The drawing under review shows one solid part. Ordinate dimensions are in mm from its lowest x, y, z. A direction names the side the tool comes from. Coordinates: 2 decimals unless noted, no trailing zeros. Order: outer loops, then holes, each group sorted by start corner. A loop starts at its lowest first (then second) coordinate and runs counter-clockwise, first axis right, second up. Notation, with made-up numbers: (39.5, 19) -> (97.5, 19) arc R32 cw to (97.5, 54) -> close; hole circle Ø1 at (-22, -30.75). An arc over 180 degrees is marked (long way). Put each result on its own line as item: value.
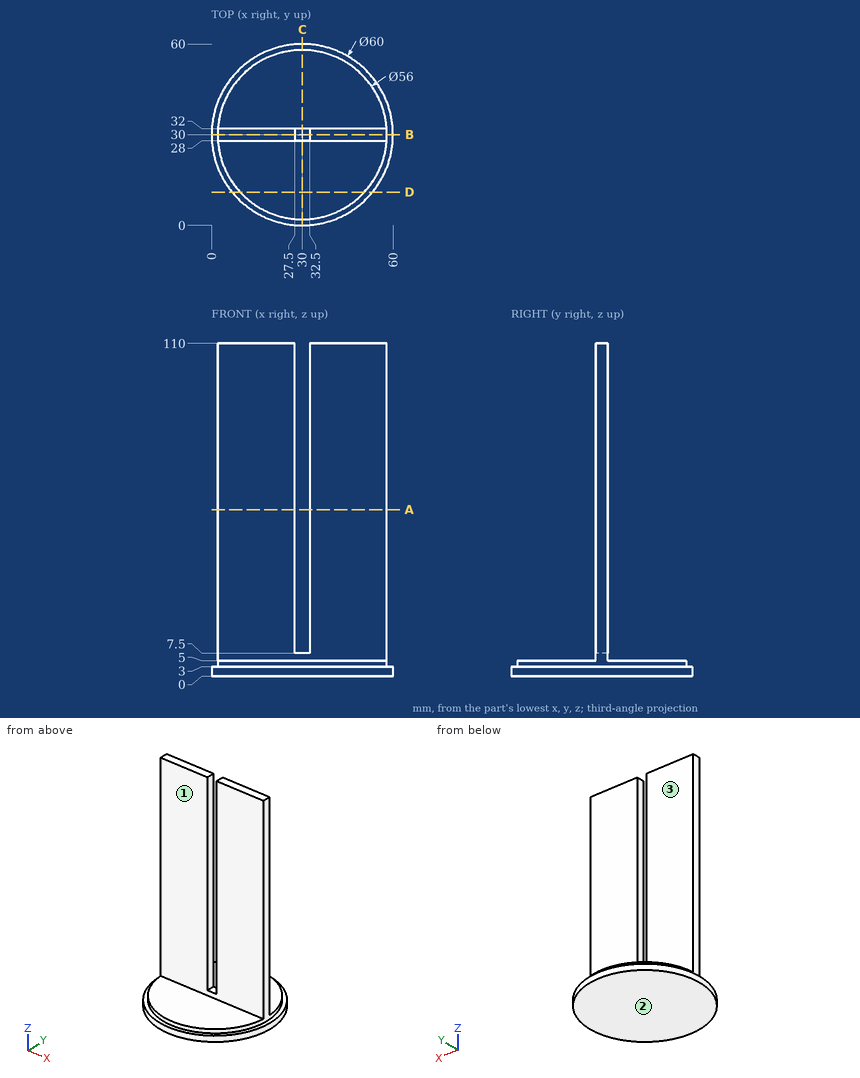
Item 1: For the marked faces 1, 2 and 3, list the 3-axis set-ups (+Z, -Z, +X, -X, +Y, -Y) from which the entire face can be reached by the end or side of a thin tool; tool diameter is ignored.
Answers below:
face 1: +Z, +X, -X, -Y
face 2: -Z, +X, -X, +Y, -Y
face 3: +Z, +X, -X, +Y
Item 2: Consider section D-D on y = 11. Write out the cut boundary in (x, z).
Answers below:
outline: (6.78, 0) -> (53.22, 0) -> (53.22, 3) -> (50.57, 3) -> (50.57, 5) -> (9.43, 5) -> (9.43, 3) -> (6.78, 3) -> close
Item 3: For line 1 (Z direction, x = 6, y = 46); line 2 (Z direction, x = 21, y = 49); line 3 (Y direction, x = 50, z = 47), list the stretches that pass through material, from the lowest coordinate up. Write a range as from..to.
Answers below:
line 1: 0..3
line 2: 0..5
line 3: 28..32
Item 4: For pin 1 Ø5 at (x, z) = (23, 58.5) entering from +Y; pin 2 Ø4.5 at (y, z) = (31, 39.5) entering from -X; pin 3 Ø1.2 at (y, z) = (30.5, 67.5) entering from +X, all flat-tipped, find the tip position at first contact; note any pin that passes through.
Answers below:
pin 1: y = 32
pin 2: x = 2
pin 3: x = 58
Item 5: Consider section A-A on z = 55. Write out the cut boundary in (x, y), and give its area (3 significant figures).
Answers below:
outline: (2.07, 28) -> (27.5, 28) -> (27.5, 32) -> (2.07, 32) arc R28 ccw to start; (32.5, 28) -> (57.93, 28) arc R28 ccw to (57.93, 32) -> (32.5, 32) -> close
area: 204 mm^2
Item 6: Consider section C-C on x = 30. Write out the cut boundary in (y, z).
Answers below:
outline: (0, 0) -> (60, 0) -> (60, 3) -> (58, 3) -> (58, 5) -> (32, 5) -> (32, 7.5) -> (28, 7.5) -> (28, 5) -> (2, 5) -> (2, 3) -> (0, 3) -> close
Item 7: Consider section B-B on y = 30. Write out the cut boundary in (x, z), and give its area (3 significant figures).
Answers below:
outline: (0, 0) -> (60, 0) -> (60, 3) -> (58, 3) -> (58, 110) -> (32.5, 110) -> (32.5, 7.5) -> (27.5, 7.5) -> (27.5, 110) -> (2, 110) -> (2, 3) -> (0, 3) -> close
area: 5,660 mm^2
